```python
from build123d import *

# Parameters (mm, degrees)
SKETCH1_W           = 16
SKETCH1_H           = 4
SKETCH1_W_2         = 2.7
SKETCH1_H_2         = 2.7
BOSS_EXTRUDE1_DEPTH = 17.1
SKETCH2_W           = 4.7
SKETCH2_H           = 1
BOSS_EXTRUDE2_DEPTH = 0.7
BOSS_EXTRUDE3_DEPTH = 1.3
SKETCH4_W           = 2.9
SKETCH4_H           = 1
BOSS_EXTRUDE4_DEPTH = 0.7


with BuildPart() as part:
    # Sketch1 → Boss-Extrude1 (new body)
    with BuildSketch(Plane(origin=(0, 0, 0), x_dir=(1, 0, 0), z_dir=(0, 1, 0))):
        Rectangle(SKETCH1_W, SKETCH1_H)
        with Locations((3, 0)):
            Rectangle(SKETCH1_W_2, SKETCH1_H_2, mode=Mode.SUBTRACT)
        Rectangle(SKETCH1_W_2, SKETCH1_H_2, mode=Mode.SUBTRACT)
        with Locations((6, 0)):
            Rectangle(SKETCH1_W_2, SKETCH1_H_2, mode=Mode.SUBTRACT)
        with Locations((-6, 0)):
            Rectangle(SKETCH1_W_2, SKETCH1_H_2, mode=Mode.SUBTRACT)
        with Locations((-3, 0)):
            Rectangle(SKETCH1_W_2, SKETCH1_H_2, mode=Mode.SUBTRACT)
    extrude(amount=BOSS_EXTRUDE1_DEPTH)

    # Sketch2 → Boss-Extrude2 (add)
    with BuildSketch(Plane.XY.offset(2)):
        Polygon((-6.15, 8.4), (-8, 8.4), (-8, 0), (-6.15, 0), (-6.15, 1), align=None)
        with Locations((-3.8, 0.5)):
            Rectangle(SKETCH2_W, SKETCH2_H)
        with Locations((3.8, 0.5)):
            Rectangle(SKETCH2_W, SKETCH2_H)
        Polygon((6.15, 1), (6.15, 0), (8, 0), (8, 8.4), (6.15, 8.4), align=None)
    extrude(amount=BOSS_EXTRUDE2_DEPTH)

    # Sketch3 → Boss-Extrude3 (add, symmetric)
    with BuildSketch(Plane(origin=(0, 0, 0), x_dir=(0, 0, -1), z_dir=(1, 0, 0))):
        Polygon((-2, 16.6), (-3, 15.6), (-3, 15.1), (-2, 15.1), align=None)
    extrude(amount=BOSS_EXTRUDE3_DEPTH, both=True)

    # Sketch4 → Boss-Extrude4 (add)
    with BuildSketch(Plane(origin=(0, 0, -2), x_dir=(-1, 0, 0), z_dir=(0, 0, -1))):
        Polygon((-1.45, 0), (-1.45, 1), (-6.15, 1), (-6.15, 8.4), (-8, 8.4), (-8, 0), align=None)
        with Locations((0, 0.5)):
            Rectangle(SKETCH4_W, SKETCH4_H)
        Polygon((6.15, 8.4), (6.15, 1), (1.45, 1), (1.45, 0), (8, 0), (8, 8.4), align=None)
    extrude(amount=BOSS_EXTRUDE4_DEPTH)


solid = part.part
```
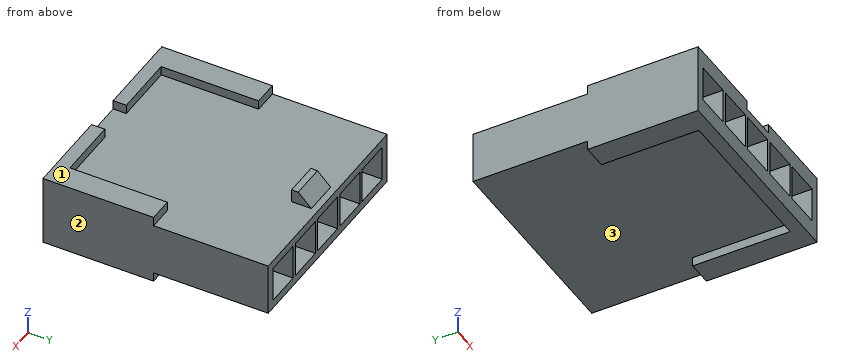
Model file for the job. Use its own axes, mm. Face numbers are marked on the shaded views. Give positions to 0.01 mm unless a question says otherwise; leave off trailing zeros. Loops run counter-clockwise (first coordinate to the right, second up) from the corner with the lowest first, then second, coordinate; pieces in that order, holes last. Notation, with made-up numbers: M 30.5,31 L 57.5,31 A9 cw 57.5,40 Z; hole C 51,86.5 d4. An arc over 180 degrees is marked long. Use one line per item in the form item = value.
Item 1: Slice it at B-B on z = -0.1. List the corners of the cut face in (x, y), and give its area (4 significant figures).
Filled in:
outline = M -8,0 L -7.35,0 L -7.35,17.1 L -8,17.1 Z; M -4.65,0 L -4.35,0 L -4.35,17.1 L -4.65,17.1 Z; M -1.65,0 L -1.35,0 L -1.35,17.1 L -1.65,17.1 Z; M 1.35,0 L 1.65,0 L 1.65,17.1 L 1.35,17.1 Z; M 4.35,0 L 4.65,0 L 4.65,17.1 L 4.35,17.1 Z; M 7.35,0 L 8,0 L 8,17.1 L 7.35,17.1 Z
area = 42.75 mm^2
Item 2: Drill centre lines: L1, parallel to X at y = 14.25, z = -0.5; L2, parallel to Z at x = -1, y = 1.5; L3, parallel to X at y = 4, z = -2.3. Where is each one in solid material? Low to high.
Filled in:
L1 = -8 to -7.35, -4.65 to -4.35, -1.65 to -1.35, 1.35 to 1.65, 4.35 to 4.65, 7.35 to 8
L2 = -2 to -1.35, 1.35 to 2
L3 = -8 to -6.15, 6.15 to 8
Item 3: Flat gauge pins, fed straight in: pin 1 Ø7 at (x, y) = (5.5, 5.5) entering from +Z; pin 2 Ø2 at (x, y) = (-6, 4.5) entering from -Z; pin 3 Ø1.5 at (x, y) = (-1, 13) entering from -Z; pin 4 Ø0.8 at (x, z) = (0.5, -2.5) entering from +Y. Where does each tip first touch, or does it go through?
Filled in:
pin_1 = 2.7
pin_2 = -2.7
pin_3 = -2
pin_4 = 1
Item 4: Slice it at C-C on x = -7. List the corners of the cut face in (y, z), and give its area (3 significant figures).
Filled in:
outline = M 0,-2.7 L 8.4,-2.7 L 8.4,-2 L 17.1,-2 L 17.1,-1.35 L 0,-1.35 Z; M 0,1.35 L 17.1,1.35 L 17.1,2 L 8.4,2 L 8.4,2.7 L 0,2.7 Z
area = 34.0 mm^2
Item 5: Two-plate mould, pull along X, no slides. Class the marked faces 1, 2 and 3: released by +X, released by -X, zero draft, split by the parting line, or undercut.
Filled in:
face_1 = zero draft
face_2 = released by +X
face_3 = undercut
Item 6: Slice it at D-D on x = -3.5. List the corners of the cut face in (y, z).
Filled in:
outline = M 0,-2.7 L 1,-2.7 L 1,-2 L 17.1,-2 L 17.1,-1.35 L 0,-1.35 Z; M 0,1.35 L 17.1,1.35 L 17.1,2 L 1,2 L 1,2.7 L 0,2.7 Z
Item 7: Slice it at A-A on y = 14.25. List the corners of the cut face in (x, z).
Filled in:
outline = M -8,-2 L 8,-2 L 8,2 L -8,2 Z; hole M -7.35,-1.35 L -4.65,-1.35 L -4.65,1.35 L -7.35,1.35 Z; hole M -4.35,-1.35 L -1.65,-1.35 L -1.65,1.35 L -4.35,1.35 Z; hole M -1.35,-1.35 L 1.35,-1.35 L 1.35,1.35 L -1.35,1.35 Z; hole M 1.65,-1.35 L 4.35,-1.35 L 4.35,1.35 L 1.65,1.35 Z; hole M 4.65,-1.35 L 7.35,-1.35 L 7.35,1.35 L 4.65,1.35 Z
